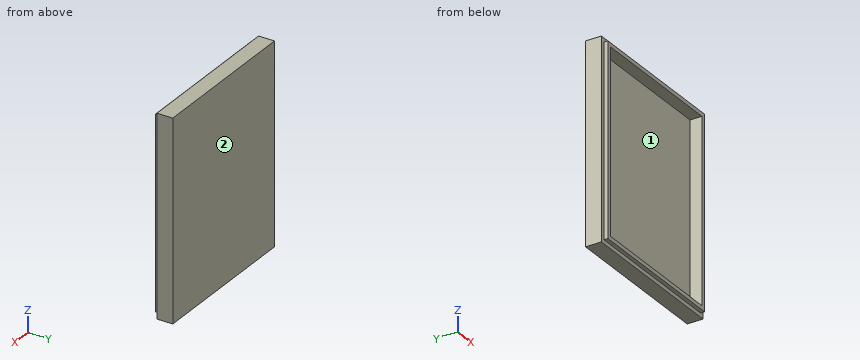
from build123d import *

# Parameters (mm, degrees)
F0_W     = 40
F0_H     = 50
F1_DEPTH = 2
F2_W     = 40
F2_H     = 50
F2_W_2   = 36
F2_H_2   = 46
F3_DEPTH = 2
F4_W     = 38
F4_H     = 48
F4_W_2   = 36
F4_H_2   = 46
F5_DEPTH = 1


with BuildPart() as f1:
    # F0 (on Front) → F1 (new body)
    with BuildSketch(Plane.XZ):
        Rectangle(F0_W, F0_H)
    extrude(amount=F1_DEPTH)

    # F2 (on face) → F3 (join)
    with BuildSketch(Plane.XZ.offset(2)):
        Rectangle(F2_W, F2_H)
        Rectangle(F2_W_2, F2_H_2, mode=Mode.SUBTRACT)
    extrude(amount=F3_DEPTH)

    # F4 (on face) → F5 (join)
    with BuildSketch(Plane.XZ.offset(4)):
        Rectangle(F4_W, F4_H)
        Rectangle(F4_W_2, F4_H_2, mode=Mode.SUBTRACT)
    extrude(amount=F5_DEPTH)


solid = f1.part
Verification items for the finished model (mm, model axes). Face numbers are marked on the shaded views. Coordinates: 2 decimals unless noted, no trailing zeros. Write each loop counter-clockwise with the first axis right and the second up, starting at its lowest first coordinate (ties: lowest second). Pieces come first, ordered by that corner, then holes. Notation, with made-up numbers: (14.25, -12.75) - (55.25, -12.75) arc R34 ccw to (55.25, 21.25) - close; hole circle Ø3 at (10, 43). An arc over 180 degrees is marked (long way). Answer as a JSON object with one key per item and string values.
(1) Mould release check, pull along Z, two halves, no side actions. Record for the marked faces 1 and 2: pulls with the +Z half, pulls with the -Z half, needs draft (parallel to the pull), parting line crosses it, or undercut.
Report:
{"face 1": "undercut", "face 2": "needs draft"}
(2) Cross-section at B-B on y = -3.2. Record the cut outline in (x, z), plus the area to 3 significant figures.
Report:
{"outline": "(-20, -25) - (20, -25) - (20, 25) - (-20, 25) - close; hole (-18, -23) - (18, -23) - (18, 23) - (-18, 23) - close", "area": "344 mm^2"}
(3) Cross-section at A-A on x = 16.5. Record the cut outline in (y, z), plus the area to 3 significant figures.
Report:
{"outline": "(-5, -24) - (-4, -24) - (-4, -25) - (0, -25) - (0, 25) - (-4, 25) - (-4, 24) - (-5, 24) - (-5, 23) - (-2, 23) - (-2, -23) - (-5, -23) - close", "area": "110 mm^2"}
(4) Gauge pin test, flat ends, axial feed: pin 1 Ø0.5 at (y, z) = (-4.5, 5) entering from -X; pin 2 Ø1 at (x, z) = (-12.5, -7.5) entering from -Y. Record the tip position at first contact, or that the pin passes through.
Report:
{"pin 1": "x = -19", "pin 2": "y = -2"}
(5) Thickness scan on line 1 along X through (y, z) = (-4.1, 13); line 2 along X through (y, z) = (-2.8, 18.5); line 3 along Y through (x, z) = (-8, -10). Record the ranges inside material, lowest first.
Report:
{"line 1": "-19 to -18, 18 to 19", "line 2": "-20 to -18, 18 to 20", "line 3": "-2 to 0"}
(6) Cross-section at C-C on z = -17. Record the cut outline in (x, y).
Report:
{"outline": "(-20, -4) - (-19, -4) - (-19, -5) - (-18, -5) - (-18, -2) - (18, -2) - (18, -5) - (19, -5) - (19, -4) - (20, -4) - (20, 0) - (-20, 0) - close"}
